Geometry: see drawing. Coordinates: mm, zero at the bounding-box minimum. A direction names the side the tool comes from. Coordinates: 2 decimals unless noted, no trailing zeros. Order: outer loops, then holes, each group sorted by start corner. A loop starts at its lowest first (then second) coordinate and runs counter-clockwise, first axis right, second up.
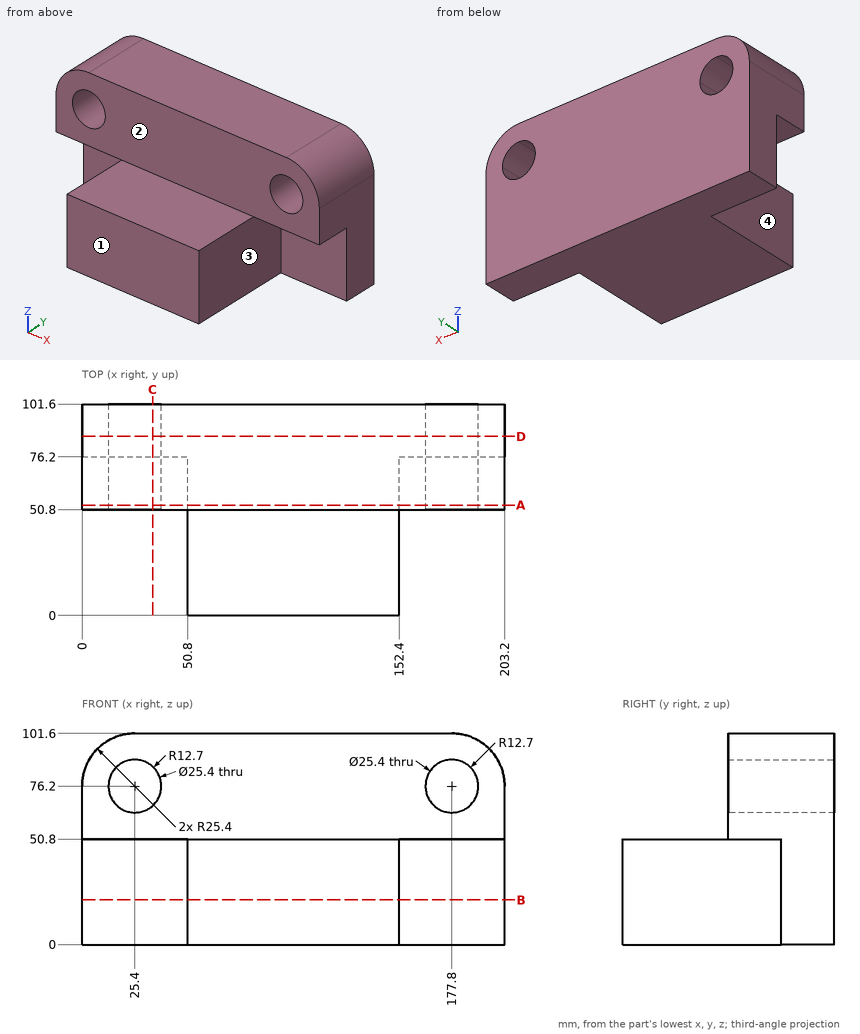
Item 1: Access query for the marked faces 1, 2, 3 and 4. Directions: +Z, -Z, +X, -X, +Y, -Y. A direction counts if a zero-diameter tool reaches every point of the face in a straight line with its end or side. Return the directions, or none.
Response values:
face 1: +Z, -Z, +X, -X, -Y
face 2: +Z, +X, -X, -Y
face 3: -Z, +X, -Y
face 4: -Z, -X, -Y
Item 2: Cut plane C-C on x = 34. Return loops of the section in (y, z).
Response values:
outline: (50.8, 50.8) - (76.2, 50.8) - (76.2, 0) - (101.6, 0) - (101.6, 66.85) - (50.8, 66.85) - close; (50.8, 85.55) - (101.6, 85.55) - (101.6, 101.6) - (50.8, 101.6) - close
Item 3: Cut plane B-B on z = 21.5. Return loops of the section in (x, y).
Response values:
outline: (0, 76.2) - (50.8, 76.2) - (50.8, 0) - (152.4, 0) - (152.4, 76.2) - (203.2, 76.2) - (203.2, 101.6) - (0, 101.6) - close
Item 4: Cut plane A-A on y = 53. Return loops of the section in (x, z).
Response values:
outline: (0, 50.8) - (50.8, 50.8) - (50.8, 0) - (152.4, 0) - (152.4, 50.8) - (203.2, 50.8) - (203.2, 76.2) arc R25.4 ccw to (177.8, 101.6) - (25.4, 101.6) arc R25.4 ccw to (0, 76.2) - close; hole circle Ø25.4 at (25.4, 76.2); hole circle Ø25.4 at (177.8, 76.2)
Item 5: Pin query (flat end, axial travel): pin 1 Ø15 at (x, y) = (78.5, 28) entering from +Z; pin 2 Ø3 at (x, y) = (73, 22.5) entering from -Z; pin 3 Ø10 at (y, z) = (14.5, 21) entering from +X; pin 4 Ø8 at (y, z) = (57, 27) entering from -X. Return the tip coordinate at first contact, or that it passes through.
Response values:
pin 1: stops at z = 50.8
pin 2: stops at z = 0
pin 3: stops at x = 152.4
pin 4: stops at x = 50.8
Item 6: Cut plane D-D on y = 86. Return loops of the section in (x, z).
Response values:
outline: (0, 0) - (203.2, 0) - (203.2, 76.2) arc R25.4 ccw to (177.8, 101.6) - (25.4, 101.6) arc R25.4 ccw to (0, 76.2) - close; hole circle Ø25.4 at (25.4, 76.2); hole circle Ø25.4 at (177.8, 76.2)
Item 7: Ray query, probe 1 along X at (y, z) = (63, 76.2); probe 2 along Z at (x, y) = (25, 75); probe 3 along Z at (x, y) = (177, 77). Return the intervals inside material, ascending.
Response values:
probe 1: x = 0 to 12.7, 38.1 to 165.1, 190.5 to 203.2
probe 2: z = 50.8 to 63.51, 88.89 to 101.6
probe 3: z = 0 to 63.53, 88.87 to 101.6
